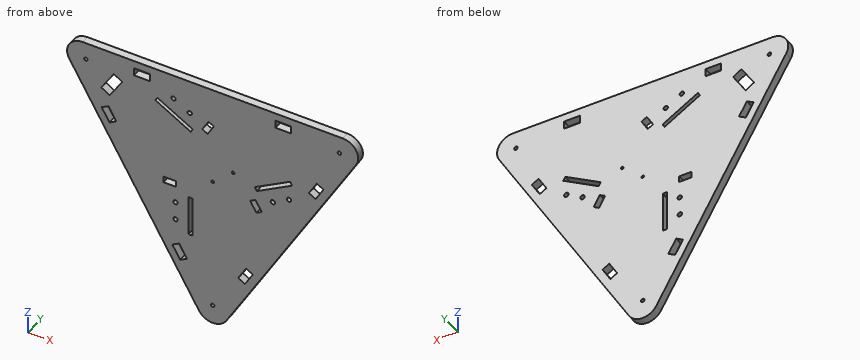
```python
from build123d import *

# Parameters (mm, degrees)
BOSS_EXTRUDE1_DEPTH = 6.35
SKETCH2_W           = 3.302
SKETCH2_H           = 33.02
SKETCH2_R           = 1.778
CUT_EXTRUDE1_DEPTH  = 195.099602868
SKETCH3_R           = 1.4224
SKETCH3_W           = 10
SKETCH3_H           = 5
CUT_EXTRUDE2_DEPTH  = 195.099602868
SKETCH4_R           = 1.0922
CUT_EXTRUDE3_DEPTH  = 195.099602868
FILLET1_R           = 12.7
SKETCH5_W           = 12.7
SKETCH5_H           = 6.35
CUT_EXTRUDE4_DEPTH  = 179.426731159
CUT_EXTRUDE5_DEPTH  = 179.426731159


with BuildPart() as part:
    # Sketch1 → Boss-Extrude1 (new body)
    with BuildSketch(Plane(origin=(0, 0, 0), x_dir=(1, 0, 0), z_dir=(0, 1, 0))):
        Polygon((0, 146.646968374), (-127, -73.323484187), (127, -73.323484187), align=None)
    extrude(amount=BOSS_EXTRUDE1_DEPTH)

    # Sketch2 → Cut-Extrude1 (cut, through all)
    with BuildSketch(Plane(origin=(0, 6.35, 0), x_dir=(1, 0, 0), z_dir=(0, 1, 0))):
        with Locations((-17.907, 46.362701567)):
            Rectangle(SKETCH2_W, SKETCH2_H)
        Polygon((64.228356761, -14.498625936), (35.632197928, 2.011374064), (33.981197928, -0.848241819), (62.577356761, -17.358241819), align=None)
        with Locations(Location((48.644716778, 6.588823684, 0), (0, 0, 270))):
            Circle(SKETCH2_R)
        with Locations(Location((61.686284992, -0.940729235, 0), (0, 0, 270))):
            Circle(SKETCH2_R)
        with Locations(Location((-30.028447081, 38.833148648, 0), (0, 0, 270))):
            Circle(SKETCH2_R)
        with Locations(Location((-30.028447081, 53.892254486, 0), (0, 0, 270))):
            Circle(SKETCH2_R)
        Polygon((-16.074197928, -31.864075631), (-17.725197928, -29.004459747), (-46.321356761, -45.514459747), (-44.670356761, -48.374075631), align=None)
        with Locations(Location((-18.616269697, -45.421972332, 0), (0, 0, 270))):
            Circle(SKETCH2_R)
        with Locations(Location((-31.657837912, -52.951525251, 0), (0, 0, 270))):
            Circle(SKETCH2_R)
    extrude(amount=-CUT_EXTRUDE1_DEPTH, mode=Mode.SUBTRACT)

    # Sketch3 → Cut-Extrude2 (cut, through all)
    with BuildSketch(Plane(origin=(0, 6.35, 0), x_dir=(1, 0, 0), z_dir=(0, 1, 0))):
        with Locations(Location((0, 118.312139176, 0), (0, 0, 270))):
            Circle(SKETCH3_R)
        with Locations(Location((-102.461318102, -59.156069588, 0), (0, 0, 270))):
            Circle(SKETCH3_R)
        with Locations(Location((102.461318102, -59.156069588, 0), (0, 0, 270))):
            Circle(SKETCH3_R)
        with Locations((-34.558, 22.352701567)):
            Rectangle(SKETCH3_W, SKETCH3_H)
        Polygon((0.935056109, -41.324967823), (-4.064943891, -32.664713785), (-8.395070909, -35.164713785), (-3.395070909, -43.824967823), align=None)
        Polygon((35.320943891, 21.472266256), (30.320943891, 12.812012218), (34.651070909, 10.312012218), (39.651070909, 18.972266256), align=None)
    extrude(amount=-CUT_EXTRUDE2_DEPTH, mode=Mode.SUBTRACT)

    # Sketch4 → Cut-Extrude3 (cut, through all)
    with BuildSketch(Plane(origin=(0, 6.35, 0), x_dir=(1, 0, 0), z_dir=(0, 1, 0))):
        with Locations(Location((0, 8.207705491, 0), (0, 0, 270))):
            Circle(SKETCH4_R)
        with Locations(Location((16.51, -6.397294509, 0), (0, 0, 270))):
            Circle(SKETCH4_R)
    extrude(amount=-CUT_EXTRUDE3_DEPTH, mode=Mode.SUBTRACT)

    # Fillet1
    fillet1_edges = [part.edges().sort_by_distance(p)[0] for p in [
        (127, 3.175, 73.323484187),
        (-127, 3.175, 73.323484187),
        (0, 3.175, -146.646968374),
    ]]
    fillet(fillet1_edges, radius=FILLET1_R)

    # Sketch5 → Cut-Extrude4 (cut, through all)
    with BuildSketch(Plane(origin=(0, 6.35, 0), x_dir=(1, 0, 0), z_dir=(0, 1, 0))):
        with Locations((-57.15, -63.798484187)):
            Rectangle(SKETCH5_W, SKETCH5_H)
        with Locations((57.15, -63.798484187)):
            Rectangle(SKETCH5_W, SKETCH5_H)
        Polygon((89.632293954, -21.300718754), (83.282293954, -10.302196126), (77.78303264, -13.477196126), (84.13303264, -24.475718754), align=None)
        Polygon((26.98303264, 74.510984899), (32.482293954, 77.685984899), (26.132293954, 88.684507527), (20.63303264, 85.509507527), align=None)
        Polygon((-26.250738686, 88.479355234), (-32.600738686, 77.480832606), (-27.101477372, 74.305832606), (-20.751477372, 85.304355234), align=None)
        Polygon((-77.901477372, -13.682348419), (-83.400738686, -10.507348419), (-89.750738686, -21.505871047), (-84.251477372, -24.680871047), align=None)
    extrude(amount=-CUT_EXTRUDE4_DEPTH, mode=Mode.SUBTRACT)

    # Sketch6 → Cut-Extrude5 (cut, through all)
    with BuildSketch(Plane(origin=(0, 6.35, 0), x_dir=(1, 0, 0), z_dir=(0, 1, 0))):
        Polygon((-73.125150775, -50.833442097), (-83.259043602, -34.761596647), (-90.026136423, -39.02849889), (-79.892243597, -55.10034434), align=None)
    extrude(amount=-CUT_EXTRUDE5_DEPTH, mode=Mode.SUBTRACT)


solid = part.part
```
The listing builds one solid part. Answer for the finished solid, in the listing's coordinates (mm). Round coordinates to 2 decimals unless told otherwise and drop trailing zeros.
Q1. Find the intervals of material crossed by line 1 (X direction, y = 1.25, z = 53); line 2 (X direction, y = 2.5, z = -54.5); line 3 (Z direction, x = -24.5, y = 3.5), in increasing order.
Q2. Given pin 1 Ø2.5 at (y, z) = (2.5, -23) entering from +X; pin 2 Ø3 at (x, z) = (-18.62, 45.42) entering from +Y; pin 3 Ø1.9 at (y, z) = (4, -44.5) entering from -X; pin 4 Ø1.5 at (y, z) = (4, -84) entering from +X, each flat-ended and moving along its own axis, determine where each tip first touches the part or whether it passes through.
Q3. Section A-A, the plane y = 4 is taken. Count the separate pieces of the cut face and the enclosed holes in it, then the cut area to 3 significant figures.
Completed:
1. line 1: x = -115.27 to -81.22, -76.56 to -33.44, -29.88 to 115.27
1. line 2: x = -53.2 to -31.7, -28.36 to -19.56, -16.26 to 53.2
1. line 3: z = -104.21 to -87.47, -78.81 to 32.92, 36.73 to 73.32
2. pin 1: stops at x = 72.11
2. pin 2: passes through
2. pin 3: stops at x = -59.52
2. pin 4: stops at x = 36.6
3. separate pieces: 1
3. enclosed holes: 24
3. area: 26,400 mm2
